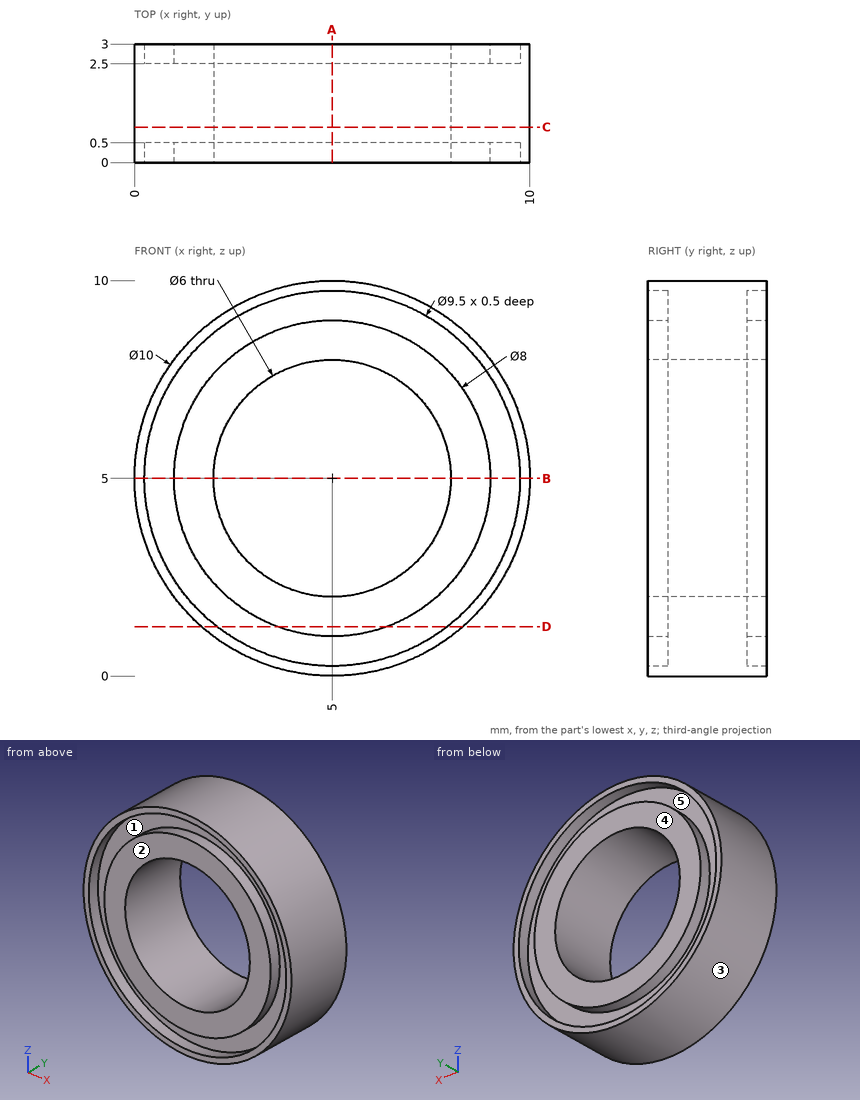
Design review of the part shown in the three views and the two pictorial views. Dimensions are in mm from the part's minimum x, y and z. A direction names the side the tool comes from. Give positions to 0.01 mm unless a question says otherwise; leave off trailing zeros. Write each loop counter-clockwise with the first axis right and the second up, starting at its lowest first coordinate (ties: lowest second). Pieces come first, ordered by that corner, then holes. Notation, with made-up numbers: M 55.5,80.25 L 96.5,80.25 A28 cw 96.5,116.25 Z; hole C 32.25,7.5 d2. An arc over 180 degrees is marked long. Return JSON: item names as keys, results as strings. Group by question number.
Item 1: Wall thickness on line 1 along X through (y, z) = (0.2, 5); line 2 along Z through (x, y) = (7.75, 0.4); line 3 along X through (y, z) = (0.2, 3.75): over which ranges is each line inside the solid? List them lowest first.
Item 2: Take a section at C-C (y = 0.9). Give the boundary of the cut face in (x, z).
Item 3: Take a section at D-D (z = 1.25). Give the boundary of the cut face in (x, y), plus the area to 3 significant figures.
Item 4: Tool access review of the marked faces 1 and 2: name each direction out of +Z, -Z, +X, -X, +Y, -Y from which nothing blocks a thin tool from reaching the whole face with its end or side.
Item 5: Take a section at A-A (x = 5). Give the boundary of the cut face in (y, z), plus the area to 3 significant figures.
Item 6: Take a section at B-B (z = 5). Give the boundary of the cut face in (x, y), plus the area to 3 significant figures.
Item 7: The part is to be moulded in two halves that separate along Z. For the marked faces 3, 4 and 5, say which applies: pulls with the +Z half, pulls with the -Z half, needs draft (parallel to the pull), parting line crosses it, or undercut.
Item 8: Clearance check with flat-ended pins moving along their axes: pin 1 Ø1.5 at (x, y) = (1, 1) entering from +Z; pin 2 Ø1 at (x, y) = (8, 2.5) entering from +Z. State where each tip first meets the part, or that it passes through.
Return value:
{
 "1": {"line 1": "x = 0 to 0.25, 1 to 2, 8 to 9, 9.75 to 10", "line 2": "z = 0.82 to 1.13, 2.1 to 3.8, 6.2 to 7.9, 8.87 to 9.18", "line 3": "x = 0.16 to 0.42, 1.2 to 2.27, 7.73 to 8.8, 9.58 to 9.84"},
 "2": {"outline": "C 5,5 d10; hole C 5,5 d6"},
 "3": {"outline": "M 1.69,0 L 2.08,0 L 2.08,0.5 L 3.61,0.5 L 3.61,0 L 6.39,0 L 6.39,0.5 L 7.92,0.5 L 7.92,0 L 8.31,0 L 8.31,3 L 7.92,3 L 7.92,2.5 L 6.39,2.5 L 6.39,3 L 3.61,3 L 3.61,2.5 L 2.08,2.5 L 2.08,3 L 1.69,3 Z", "area": "16.8 mm2"},
 "4": {"face 1": "-Y", "face 2": "+Z, -Z, +X, -X, -Y"},
 "5": {"outline": "M 0,0 L 3,0 L 3,0.25 L 2.5,0.25 L 2.5,1 L 3,1 L 3,2 L 0,2 L 0,1 L 0.5,1 L 0.5,0.25 L 0,0.25 Z; M 0,8 L 3,8 L 3,9 L 2.5,9 L 2.5,9.75 L 3,9.75 L 3,10 L 0,10 L 0,9.75 L 0.5,9.75 L 0.5,9 L 0,9 Z", "area": "10.5 mm2"},
 "6": {"outline": "M 0,0 L 0.25,0 L 0.25,0.5 L 1,0.5 L 1,0 L 2,0 L 2,3 L 1,3 L 1,2.5 L 0.25,2.5 L 0.25,3 L 0,3 Z; M 8,0 L 9,0 L 9,0.5 L 9.75,0.5 L 9.75,0 L 10,0 L 10,3 L 9.75,3 L 9.75,2.5 L 9,2.5 L 9,3 L 8,3 Z", "area": "10.5 mm2"},
 "7": {"face 3": "parting line crosses it", "face 4": "needs draft", "face 5": "undercut"},
 "8": {"pin 1": "stops at z = 8.8", "pin 2": "stops at z = 9.33"}
}
